Can you work these out from the model? Positions are in its coordinate system, mm. A direction names the side the tool comes from. Coordinates: 2 decimals unless noted, no trailing zeros. Use one line per item in the form item = value. Start each with the question number.
(1) For pin 1 Ø12 at (x, y) = (5.5, 29.5) entering from +Z; pin 2 Ø12 at (x, y) = (39.5, 38) entering from +Z, each with a flat end and sliding along its axis, tell me the tip position at first contact or that it passes through.
(2) If I drill on probe 1 along Z at (x, y) = (38, 22); probe 2 along X at (y, z) = (31.5, 24); probe 3 along Y at (x, z) = (-45.5, -39.5), over which ranges is the centre line in solid material (lowest first)? Write a range as from..to.
(3) On a 3-axis mill with a long thin cutter (end or side, diameter ignored), from which of +Z, -Z, +X, -X, +Y, -Y can I reach the whole of each face in a straight line? I mean faces 1 (the face through (27, 27, 55.372)), 2 (the face through (-54.633, 27, 28)), 3 (the face through (-27, -0.363, 29)), 4 (the face through (12, 0, -17)). Say none if no direction works.
```python
from build123d import *

# Parameters (mm, degrees)
F0_W     = 52.9774986207
F0_H     = 61.4581517875
F1_DEPTH = 55.372
F2_W     = 54.633140564
F2_H     = 56.3007220626
F3_DEPTH = 53.34
F4_W     = 52.9774986207
F4_H     = 61.4581517875
F5_DEPTH = 55.372
F6_W     = 55.372
F6_H     = 52.9774986207
F7_DEPTH = 55.372


with BuildPart() as f1:
    # F0 (on Right) → F1 (new body)
    with BuildSketch(Plane.YZ):
        with Locations((26.4887493104, -30.7290758938)):
            Rectangle(F0_W, F0_H)
    extrude(amount=-F1_DEPTH)

    # F2 (on face) → F3 (join)
    with BuildSketch(Plane(origin=(0, 52.9774986207, 0), x_dir=(-1, 0, 0), z_dir=(0, 1, 0))):
        with Locations((27.316570282, 28.1503610313)):
            Rectangle(F2_W, F2_H)
    extrude(amount=-F3_DEPTH)

    # F4 (on face) → F5 (join)
    with BuildSketch(Plane.YZ):
        with Locations((26.4887493104, -30.7290758938)):
            Rectangle(F4_W, F4_H)
    extrude(amount=F5_DEPTH)

    # F6 (on face) → F7 (join)
    with BuildSketch(Plane.XY):
        with Locations((27.686, 26.4887493104)):
            Rectangle(F6_W, F6_H)
    extrude(amount=F7_DEPTH)


solid = f1.part
```
Reported:
q1.pin_1 = 56.3
q1.pin_2 = 55.37
q2.probe_1 = -61.46..55.37
q2.probe_2 = -54.63..55.37
q2.probe_3 = 0..52.98
q3.face_1 = +Z, +X, +Y, -Y
q3.face_2 = +Z, -X, +Y, -Y
q3.face_3 = +Z, -Z, +X, -X, -Y
q3.face_4 = -Z, +X, -Y
